from build123d import *

# Parameters (mm, degrees)
SKETCH1_W           = 25.4
SKETCH1_H           = 127
SKETCH1_R           = 3.175
BOSS_EXTRUDE1_DEPTH = 25.4
BOSS_EXTRUDE2_DEPTH = 25.4
BOSS_EXTRUDE3_DEPTH = 12.7
BOSS_EXTRUDE4_DEPTH = 12.7
SKETCH5_R           = 3.175
CUT_EXTRUDE1_DEPTH  = 96.25
SKETCH6_R           = 5.08
CUT_EXTRUDE2_DEPTH  = 76.2


with BuildPart() as part:
    # Sketch1 → Boss-Extrude1 (new body)
    with BuildSketch(Plane.XY):
        Rectangle(SKETCH1_W, SKETCH1_H)
        with Locations((0, 50.732762061)):
            Circle(SKETCH1_R, mode=Mode.SUBTRACT)
        Circle(SKETCH1_R, mode=Mode.SUBTRACT)
        with Locations((0, -50.8)):
            Circle(SKETCH1_R, mode=Mode.SUBTRACT)
    extrude(amount=BOSS_EXTRUDE1_DEPTH)

    # Sketch2 → Boss-Extrude2 (add)
    with BuildSketch(Plane.XY.offset(25.4)):
        with BuildLine():
            Line((12.7, 63.5), (12.7, -63.5))
            Line((12.7, -63.5), (82.55, -63.5))
            Line((82.55, -63.5), (82.55, -50.8))
            ThreePointArc((82.55, -50.8), (31.75, 0), (82.55, 50.8))
            Line((82.55, 50.8), (82.55, 63.5))
            Line((82.55, 63.5), (12.7, 63.5))
        make_face()
    extrude(amount=-BOSS_EXTRUDE2_DEPTH)

    # Sketch3 → Boss-Extrude3 (add)
    with BuildSketch(Plane.XY.offset(25.4)):
        with BuildLine():
            Line((82.55, 63.5), (82.55, 50.8))
            ThreePointArc((82.55, 50.8), (31.75, 0), (82.55, -50.8))
            Line((82.55, -50.8), (82.55, -63.5))
            ThreePointArc((82.55, -63.5), (19.05, 0), (82.55, 63.5))
        make_face()
    extrude(amount=BOSS_EXTRUDE3_DEPTH)

    # Sketch4 → Boss-Extrude4 (add)
    with BuildSketch(Plane(origin=(0, 0, 0), x_dir=(-1, 0, 0), z_dir=(0, 0, -1))):
        with BuildLine():
            Line((-82.55, 63.5), (-82.55, 50.8))
            ThreePointArc((-82.55, 50.8), (-31.75, 0), (-82.55, -50.8))
            Line((-82.55, -50.8), (-82.55, -63.5))
            ThreePointArc((-82.55, -63.5), (-19.05, 0), (-82.55, 63.5))
        make_face()
    extrude(amount=BOSS_EXTRUDE4_DEPTH)

    # Sketch5 → Cut-Extrude1 (cut, through all)
    with BuildSketch(Plane(origin=(82.55, 0, 0), x_dir=(0, 0, -1), z_dir=(1, 0, 0))):
        with Locations((-31.75, 57.15)):
            Circle(SKETCH5_R)
        with Locations((6.35, 57.15)):
            Circle(SKETCH5_R)
        with Locations((6.35, -57.15)):
            Circle(SKETCH5_R)
        with Locations((-31.75, -57.15)):
            Circle(SKETCH5_R)
    extrude(amount=-CUT_EXTRUDE1_DEPTH, mode=Mode.SUBTRACT)

    # Sketch6 → Cut-Extrude2 (cut)
    with BuildSketch(Plane.ZY.offset(12.7)):
        with Locations((-6.35, 57.15)):
            Circle(SKETCH6_R)
        with Locations((31.75, 57.15)):
            Circle(SKETCH6_R)
        with Locations((31.75, -57.15)):
            Circle(SKETCH6_R)
        with Locations((-6.35, -57.15)):
            Circle(SKETCH6_R)
    extrude(amount=-CUT_EXTRUDE2_DEPTH, mode=Mode.SUBTRACT)


solid = part.part
Design review of the part built by this model. Coordinates are the model's own, in mm. A direction names the side the tool comes from. Round coordinates to 2 decimals unless told otherwise and drop trailing zeros. Loops run counter-clockwise (first coordinate to the right, second up) from the corner with the lowest first, then second, coordinate; pieces in that order, holes last. Notation, with made-up numbers: (42.5, 65.5) -> (91.5, 65.5) arc R21 cw to (91.5, 69.5) -> close; hole circle Ø1 at (74, -32). An arc over 180 degrees is marked (long way). Use one line per item in the form item = value. Start each with the question number.
Q1. Wall thickness on line 1 along Z through (x, y) = (57, 57.15); line 2 along Z through (x, y) = (21.5, 28.5); line 3 along Y through (x, z) = (63, 27.5): over which ranges is each line inside the solid? List them lowest first. Write a range as [from, to].
Q2. Machinability: for faces 4 (the face through (19.065, -1.396, 31.661)), 5 (the face through (13, 1, 0)), 6 (the face through (63.5, -53, -6)), which of the approach directions +Z, -Z, +X, -X, +Y, -Y give a long, thin tool a straight path to every point of the face, cutting with its end or side? Answer none if there is none.
Q3. We need section A-A on y = 0. Give the boundary of the cut face in (x, z) (3 decimals), then the cut area to 3 significant figures.
Q4. We need section B-B on x = 0. Give the boundary of the cut face in (y, z) (3 decimals), then the cut area to 3 significant figures.
Q5. We need section D-D on x = 59.5. Give the boundary of the cut face in (y, z).
Q6. For pin 1 Ø4 at (y, z) = (-14, -7) entering from -X; pin 2 Ø5.5 at (y, z) = (-57.15, -6.35) entering from -X; pin 3 Ø4.5 at (y, z) = (54.5, -6) entering from -X; pin 4 Ø11.5 at (y, z) = (57.15, 31.75) entering from -X, all flat-tipped, find the tip position at first contact; note any pin that passes through.
Q7. Draft analysis for pull direction Z (two halves, no side actions). For faces 1 (the face through (-0.688, 47.633, 12.522)), 2 (the face through (13, 1, 25.4)), 3 (the face through (73.16, 54.05, -5.66)), state which applies: +Z half, -Z half, draft (parallel to the pull), parting line (faces both ways), or undercut.
Q8. We need section C-C on z = 31.75. Give the boundary of the cut face in (x, y) (3 decimals), then the cut area to 3 significant figures.
Calculated:
q1.line_1 = [-12.7, -11.43], [-1.27, 26.67], [36.83, 38.1]
q1.line_2 = [0, 25.4]
q1.line_3 = [-60.42, -59.93], [-54.37, -46.89], [46.89, 54.37], [59.93, 60.42]
q2.face_4 = +Z, -X
q2.face_5 = -Z, -X
q2.face_6 = -X
q3.outline = (-12.7, 0) -> (-3.175, 0) -> (-3.175, 25.4) -> (-12.7, 25.4) -> close; (3.175, 0) -> (19.05, 0) -> (19.05, -12.7) -> (31.75, -12.7) -> (31.75, 38.1) -> (19.05, 38.1) -> (19.05, 25.4) -> (3.175, 25.4) -> close
q3.area = 1,290 mm²
q4.outline = (-63.5, 0) -> (-53.975, 0) -> (-53.975, 25.4) -> (-63.5, 25.4) -> close; (-47.625, 0) -> (-3.175, 0) -> (-3.175, 25.4) -> (-47.625, 25.4) -> close; (3.175, 0) -> (47.558, 0) -> (47.558, 25.4) -> (3.175, 25.4) -> close; (53.908, 0) -> (63.5, 0) -> (63.5, 25.4) -> (53.908, 25.4) -> close
q4.area = 2,740 mm²
q5.outline = (-63.5, 0) -> (-59.17, 0) -> (-59.17, -1.69) arc R5.08 cw (long way) to (-59.17, -11.01) -> (-59.17, -12.7) -> (-45.27, -12.7) -> (-45.27, 38.1) -> (-59.17, 38.1) -> (-59.17, 36.41) arc R5.08 cw (long way) to (-59.17, 27.09) -> (-59.17, 25.4) -> (-63.5, 25.4) -> close; (45.27, -12.7) -> (59.17, -12.7) -> (59.17, -11.01) arc R5.08 cw (long way) to (59.17, -1.69) -> (59.17, 0) -> (63.5, 0) -> (63.5, 25.4) -> (59.17, 25.4) -> (59.17, 27.09) arc R5.08 cw (long way) to (59.17, 36.41) -> (59.17, 38.1) -> (45.27, 38.1) -> close
q6.pin_1 = 20.19
q6.pin_2 = through
q6.pin_3 = 63.5
q6.pin_4 = 45.26
q7.face_1 = draft
q7.face_2 = +Z half
q7.face_3 = undercut
q8.outline = (46.205, -52.07) -> (63.5, -52.07) -> (63.5, -53.975) -> (82.55, -53.975) -> (82.55, -50.8) arc R50.8 cw to (82.55, 50.8) -> (82.55, 53.975) -> (63.5, 53.975) -> (63.5, 52.07) -> (46.205, 52.07) arc R63.5 ccw to start; (63.5, -60.575) arc R63.5 ccw to (82.55, -63.5) -> (82.55, -60.325) -> (63.5, -60.325) -> close; (63.5, 60.325) -> (82.55, 60.325) -> (82.55, 63.5) arc R63.5 ccw to (63.5, 60.575) -> close
q8.area = 1,870 mm²
